```python
from build123d import *

# Parameters (mm, degrees)
SKETCH1_R           = 7
SKETCH1_R_2         = 2.5
BOSS_EXTRUDE1_DEPTH = 21.5
SKETCH2_R           = 7.5
CUT_EXTRUDE1_DEPTH  = 1
CUT_EXTRUDE2_START  = -1
SKETCH3_R           = 7.5
CUT_EXTRUDE2_DEPTH  = 1
SKETCH5_W           = 50.8
SKETCH5_H           = 25.4
SKETCH5_W_2         = 46.5
SKETCH5_H_2         = 21.5
BOSS_EXTRUDE2_DEPTH = 5


with BuildPart() as part:
    # Sketch1 → Boss-Extrude1 (new body)
    with BuildSketch(Plane.XY):
        with BuildLine():
            Line((-23.25, 0), (-23.25, 100))
            Line((-23.25, 100), (23.25, 100))
            Line((23.25, 100), (23.25, 0))
            ThreePointArc((23.25, 0), (0, -23.25), (-23.25, 0))
        make_face()
        Circle(SKETCH1_R, mode=Mode.SUBTRACT)
        with Locations((-11.25, 85)):
            Circle(SKETCH1_R_2, mode=Mode.SUBTRACT)
        with Locations((11.25, 85)):
            Circle(SKETCH1_R_2, mode=Mode.SUBTRACT)
        with Locations((11.25, 50)):
            Circle(SKETCH1_R_2, mode=Mode.SUBTRACT)
        with Locations((-11.25, 50)):
            Circle(SKETCH1_R_2, mode=Mode.SUBTRACT)
    extrude(amount=BOSS_EXTRUDE1_DEPTH)

    # Sketch2 → Cut-Extrude1 (cut)
    with BuildSketch(Plane.XY.offset(21.5)):
        Circle(SKETCH2_R)
    extrude(amount=-CUT_EXTRUDE1_DEPTH, mode=Mode.SUBTRACT)

    # Sketch3 → Cut-Extrude2 (cut)
    with BuildSketch(Plane(origin=(0, 0, 0), x_dir=(-1, 0, 0), z_dir=(0, 0, -1)).offset(CUT_EXTRUDE2_START)):
        with Locations(Location((0, 0, 0), (0, 0, 180))):
            Circle(SKETCH3_R)
    extrude(amount=CUT_EXTRUDE2_DEPTH, mode=Mode.SUBTRACT)

    # Sketch5 → Boss-Extrude2 (add)
    with BuildSketch(Plane(origin=(0, 24.981, 0), x_dir=(1, 0, 0), z_dir=(0, 1, 0))):
        with Locations((0, -10.75)):
            Rectangle(SKETCH5_W, SKETCH5_H)
        with Locations((0, -10.75)):
            Rectangle(SKETCH5_W_2, SKETCH5_H_2, mode=Mode.SUBTRACT)
    extrude(amount=-BOSS_EXTRUDE2_DEPTH)


solid = part.part
```
Model file for the job. Use its own axes, mm. A direction names the side the tool comes from. Give positions to 0.01 mm unless a question says otherwise; leave off trailing zeros. Loops run counter-clockwise (first coordinate to the right, second up) from the corner with the lowest first, then second, coordinate; pieces in that order, holes last. Notation, with made-up numbers: M -30,-29.75 L 13,-29.75 A12 cw 13,-17.75 Z; hole C -16,3 d6. An arc over 180 degrees is marked long. Use one line per item in the form item = value.
Item 1: Slice it at C-C on z = 2.5. List the corners of the cut face in (x, y), and give its area (3 significant figures).
Filled in:
outline = M -25.4,19.98 L -23.25,19.98 L -23.25,0 A23.25 ccw 23.25,0 L 23.25,19.98 L 25.4,19.98 L 25.4,24.98 L 23.25,24.98 L 23.25,100 L -23.25,100 L -23.25,24.98 L -25.4,24.98 Z; hole C -11.25,50 d5; hole C -11.25,85 d5; hole C 0,0 d14; hole C 11.25,50 d5; hole C 11.25,85 d5
area = 5,290 mm^2
Item 2: Which spindle directions (+Z, -Z, +X, -X, +Y, -Y) get a long thin tool onto all of the face, cutting with end or side? Do faces 1 (the flat face through (23.25, 10, 11)), 2 (the flat face through (0, 63, 0)), 3 (the cylindrical face through (-7.493, 0.33, 21.007)), 4 (the flat face through (-5, -6, 0)). Say none if no direction does.
Filled in:
face_1 = +Z, -Z, +X, -Y
face_2 = -Z, +X, -X, +Y
face_3 = +Z
face_4 = -Z, +X, -X, -Y
Item 3: Slice it at B-B on x = 0. List the corners of the cut face in (y, z).
Filled in:
outline = M -23.25,0 L -7.5,0 L -7.5,1 L -7,1 L -7,20.5 L -7.5,20.5 L -7.5,21.5 L -23.25,21.5 Z; M 7,1 L 7.5,1 L 7.5,0 L 19.98,0 L 19.98,-1.95 L 24.98,-1.95 L 24.98,0 L 100,0 L 100,21.5 L 24.98,21.5 L 24.98,23.45 L 19.98,23.45 L 19.98,21.5 L 7.5,21.5 L 7.5,20.5 L 7,20.5 Z
Item 4: Flat gauge pins, fed straight in: pin 1 Ø7.5 at (x, z) = (10.5, 11) entering from -Y; pin 2 Ø23 at (x, y) = (-2, 61) entering from -Z; pin 3 Ø12 at (x, y) = (0, 0) entering from -Z; pin 4 Ø12 at (x, y) = (-0.5, -3.5) entering from +Z. Where does each tip first touch, or does it go through?
Filled in:
pin_1 = -22.25
pin_2 = 0
pin_3 = through
pin_4 = 21.5
Item 5: Slice it at D-D on x = -11.25. List the corners of the cut face in (y, z).
Filled in:
outline = M -20.35,0 L 19.98,0 L 19.98,-1.95 L 24.98,-1.95 L 24.98,0 L 47.5,0 L 47.5,21.5 L 24.98,21.5 L 24.98,23.45 L 19.98,23.45 L 19.98,21.5 L -20.35,21.5 Z; M 52.5,0 L 82.5,0 L 82.5,21.5 L 52.5,21.5 Z; M 87.5,0 L 100,0 L 100,21.5 L 87.5,21.5 Z
Item 6: Slice it at A-A on y = 85. List the corners of the cut face in (x, z).
Filled in:
outline = M -23.25,0 L -13.75,0 L -13.75,21.5 L -23.25,21.5 Z; M -8.75,0 L 8.75,0 L 8.75,21.5 L -8.75,21.5 Z; M 13.75,0 L 23.25,0 L 23.25,21.5 L 13.75,21.5 Z
Item 7: Drill centre lines: L1, parallel to Y at x = -11.5, z = 11; L2, parallel to X at y = 49, z = 9.5; L3, parallel to Y at x = -11.25, z = 6.75. Where is each one in solid material? Low to high.
Filled in:
L1 = -20.21 to 47.51, 52.49 to 82.51, 87.49 to 100
L2 = -23.25 to -13.54, -8.96 to 8.96, 13.54 to 23.25
L3 = -20.35 to 47.5, 52.5 to 82.5, 87.5 to 100
Item 8: Two-plate mould, pull along X, no slides. Class faces 5 (the cylindrical face through (9.41, 51.69, 10.6)), 6 (the flat face through (-25.4, 23, 11)), 7 (the flat face through (23.25, 63, 11)), 8 (the flat face through (-2, 24.981, 22)): released by +X, released by -X, zero draft, split by the parting line, or undercut.
Filled in:
face_5 = undercut
face_6 = released by -X
face_7 = released by +X
face_8 = zero draft
